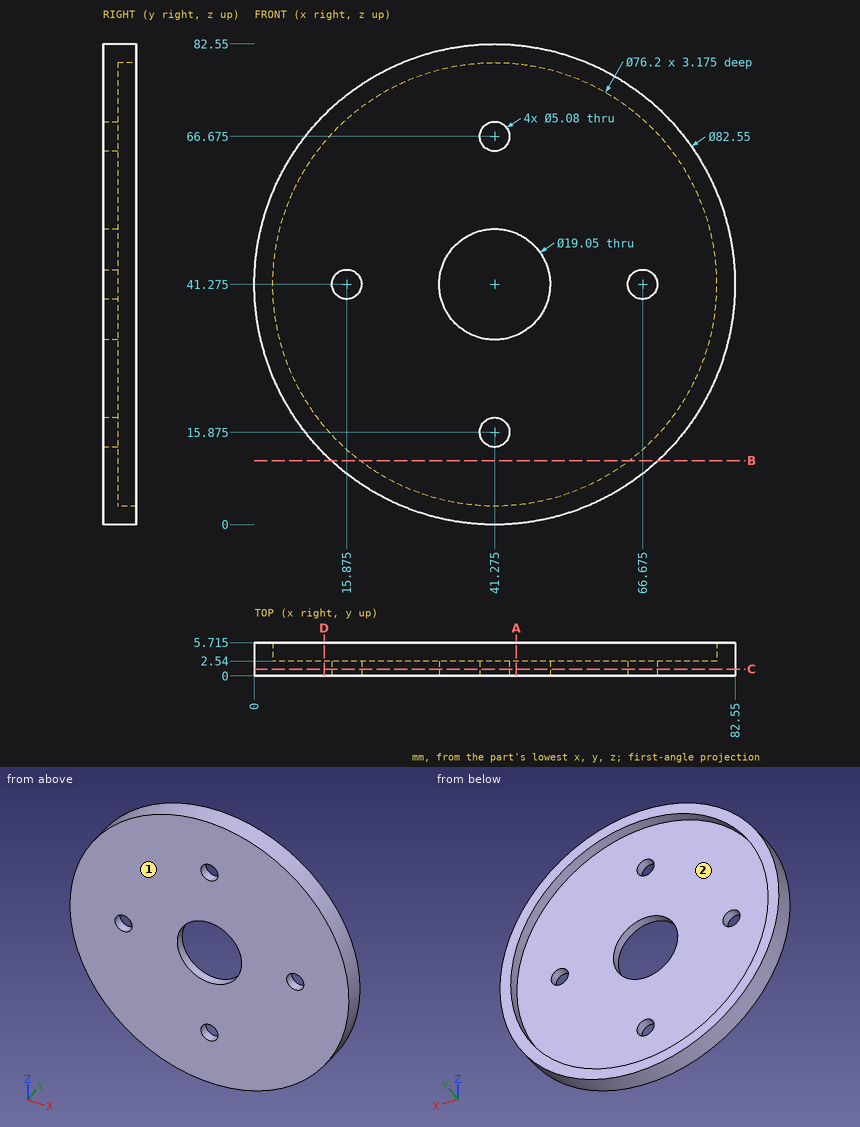
For this review, use the dimensioned drawing (mm, ordinates from the lowest corner) and the shaded views. Coordinates: 2 decimals unless noted, no trailing zeros. Loops run counter-clockwise (first coordinate to the right, second up) from the corner with the lowest first, then second, coordinate; pieces in that order, holes last. Notation, with made-up numbers: (13, 45) - (51, 45) arc R18 cw to (51, 79) - close; hole circle Ø1 at (84, 7.25). An arc over 180 degrees is marked (long way). Use one line per item in the form item = value. Start each with the question number.
1) Take a section at D-D (x = 12). State the section outline as (y, z) points (3 decimals).
2) To check wall thickness, follow probe 1 along Y at (x, z) = (11.5, 64); probe 2 along Z at (x, y) = (67, 1.6); probe 3 along X at (y, z) = (0.3, 48.5). State the ranges of each line that lie inside material, in increasing order. Write a range as from..to.
3) Take a section at C-C (y = 1.2). State the section outline as (x, z) points (3 decimals), plus the area to 3 significant figures.
4) Take a section at B-B (z = 11). State the section outline as (x, y) points (3 decimals), plus the area to 3 significant figures.
5) For pin 1 (1.5 mm diameter, centred on x = 32.5, y = 4.5, fed in from +Z); pin 2 (4 mm diameter, centred on x = 66.675, z = 41.275, fed in from -Y); pin 3 (22 mm diameter, centred on x = 41.275, z = 41.275, fed in from +Y); pin 4 (1 mm diameter, centred on x = 34.5, y = 3, fed in from +Z), all flat-tipped, find the tip position at first contact; note any pin that passes through.
6) Draft analysis for pull direction Z (two halves, no side actions). For the marked faces 1 and 2, state which applies: released by +Z, released by -Z, zero draft, split by the parting line, or undercut.
7) Take a section at A-A (x = 45). State the section outline as (y, z) points (3 decimals), plus the area to 3 significant figures.
From the geometry:
q1.outline = (0, 12.179) - (5.715, 12.179) - (5.715, 16.891) - (2.54, 16.891) - (2.54, 65.659) - (5.715, 65.659) - (5.715, 70.371) - (0, 70.371) - close
q2.probe_1 = 0..2.54
q2.probe_2 = 9..38.76, 43.79..73.55
q2.probe_3 = 0.64..35.07, 47.48..81.91
q3.outline = circle Ø82.55 at (41.275, 41.275); hole circle Ø5.08 at (15.875, 41.275); hole circle Ø19.05 at (41.275, 41.275); hole circle Ø5.08 at (41.275, 15.875); hole circle Ø5.08 at (41.275, 66.675); hole circle Ø5.08 at (66.675, 41.275)
q3.area = 4,990 mm2
q4.outline = (13.221, 0) - (69.329, 0) - (69.329, 5.715) - (64.406, 5.715) - (64.406, 2.54) - (18.144, 2.54) - (18.144, 5.715) - (13.221, 5.715) - close
q4.area = 174 mm2
q5.pin_1 = 81.76
q5.pin_2 = through
q5.pin_3 = 2.54
q5.pin_4 = 82.07
q6.face_1 = zero draft
q6.face_2 = undercut
q7.outline = (0, 0.168) - (5.715, 0.168) - (5.715, 3.358) - (2.54, 3.358) - (2.54, 32.509) - (0, 32.509) - close; (0, 50.041) - (2.54, 50.041) - (2.54, 79.192) - (5.715, 79.192) - (5.715, 82.382) - (0, 82.382) - close
q7.area = 185 mm2
